For this review, take the finished solid that the model builds, in its own axes (mm). A direction names the side the tool comes from. Coordinates: 2 decimals unless noted, no trailing zeros. Loops run counter-clockwise (first coordinate to the right, second up) from the corner with the lowest first, then second, coordinate; pieces in that order, holes last.
Autodesk Inventor part; units mm, degrees
ref_plane "YZ Plane" through (0, 0, 0) normal (1, 0, 0) x (0, 1, 0)
ref_plane "XZ Plane" through (0, 0, 0) normal (0, 1, 0) x (-1, 0, 0)
ref_plane "XY Plane" through (0, 0, 0) normal (0, 0, 1) x (1, 0, 0)
sketch "スケッチ1" plane through (0, 0, 0) normal (1, 0, 0) x (0, 1, 0)
  circle A0 centre (0, 0) radius 5
  line L0 (5, 24) -> (-10, 24)
  line L1 (-10, 24) -> (-10, 9)
  line L2 (-10, 9) -> (5, 9)
  line L3 (5, 9) -> (5, 24)
  line L4 (-10, 9) -> (-15, 9)
  line L5 (-15, 9) -> (-15, -9)
  line L6 (-15, -9) -> (-10, -9)
  line L7 (-10, -9) -> (-10, 9)
  line L8 (-10, 9) -> (1.724, 4.6934)
  line L9 (1.724, -4.6934) -> (-10, -9)
  circle A1 centre (0, 0) radius 1.6
  line L10 (-10, 9) -> (-5, 9)
  line L11 (-5, 9) -> (-5, -9)
  line L12 (-5, -9) -> (-10, -9)
  line L13 (-10, -9) -> (-10, 9)
  line L14 (-5, 9) -> (2.6415, 4.2453)
  line L15 (-5, -9) -> (2.6415, -4.2453)
  line L16 (-5, 7) -> (-10, 7)
  line L17 (-5, 7) -> (1.6216, 4.7297)
  dimension "d0" = 10
  dimension "d1" = 15
  dimension "d2" = 15
  dimension "d3" = 5
  dimension "d5" = 18
  dimension "d6" = 3.2
  dimension "d7" = 10
  dimension "d8" = 9
  dimension "d11" = 5
  dimension "d12" = 18
  dimension "d29" = 2
extrude "押し出し2" add sketch "スケッチ1" along normal blind 5 contours A0 | A0 L8 L11 L14 | L15 L11 L9 A0 | L11 L8 L2 | L9 L11 A0 | L12 L9 L11 | L17 L11 L8 | A0 L11 L17 | L8 L11 L16 L7 | L11 L9 L7 L16
fillet "フィレット1" radius 2 2 edges at (2.5, -5, -9) (2.5, -5, 9)
sketch "スケッチ2" plane through (0, -10, -9) normal (0, -1, 0) x (1, 0, 0)
  circle A0 centre (2.5, 3.5) radius 1.25
  line L0 (0, 0) -> (5, 0)
  line L1 (0, 18) -> (0, 0)
  circle A1 centre (2.5, 10.5) radius 1.25
  point P0 (0, 9)
  dimension "d16" = 2.5
  dimension "d17" = 3.5
  dimension "d18" = 2.5
  dimension "d19" = 2.5
  dimension "d20" = 2.5
  dimension "d21" = 7
hole "穴1" at (2.5, -10, 1.5) at (2.5, -10, -5.5) direction (0, 1, 0) diameter 2.5 depth 5 tip angle 118
extrude "押し出し3" cut sketch "スケッチ1" along normal blind 10 contours A0 L8 L11 L14 | L11 L8 L2 | L17 L11 L8 | L8 L11 L16 L7
fillet "フィレット2" radius 2 1 edges at (2.5, -5, 7)
equation "\"d12\" = d5"
equation "\"d18\" = d16"
equation "\"d20\" = d18"
properties part number "belt_liner_v5_Plate_10" material "アルミニウム 6061"
Q1. Machinability: for faces 1 (the face through (2.45, -7.46, -4.25)), 2 (the face through (2, -8, 7)), which of the approach directions +Z, -Z, +X, -X, +Y, -Y give a long, thin tool a straight path to every point of the face, cutting with its end or side? Answer none if there is none.
Q2. Consider section A-A (z = 0). State the section outline as (x, y) points, then the cut area to 3 significant figures.
Q3. Consider section D-D (y = 0). State the section outline as (x, z) points.
Q4. For pin 1 Ø2 at (x, y) = (3, -3) entering from -Z; pin 2 Ø2 at (x, z) = (2.5, -5.5) entering from +Y; pin 3 Ø1 at (x, y) = (4.5, 3) entering from -Z; pin 4 Ø3 at (y, z) = (0, 0) entering from +X, all flat-tipped, find the tip position at first contact; note any pin that passes through.
Q5. Consider section B-B (x = 4.1). State the section outline as (y, z) points.
Q6. Wall thickness on probe 1 along Z at (x, y) = (2.5, -7.95); probe 2 along X at (y, z) = (-8, -5.5); probe 3 along Z at (x, y) = (3.2, -8): over which ranges is each line inside the solid? List them lowest first.
Q7. The part is to be moulded in two halves that separate along Y. For faces 3 (the face through (2.465, -0.987, -6.503)), 4 (the face through (2.12, -7.46, 0.31)), 5 (the face through (2.46, -1.27, 0.97)), say which applies: +Y half, -Y half, draft (parallel to the pull), parting line (faces both ways), or undercut.
Q8. Consider section C-C (y = -6). State the section outline as (x, z) points.
Model answer:
1. face 1: -Y
1. face 2: +Z, +X, -X, +Y, -Y
2. outline: (0, -10) - (5, -10) - (5, -1.6) - (0, -1.6) - close; (0, 1.6) - (5, 1.6) - (5, 5) - (0, 5) - close
2. area: 59.0 mm2
3. outline: (0, -5.89) - (5, -5.89) - (5, -1.6) - (0, -1.6) - close; (0, 1.6) - (5, 1.6) - (5, 5.29) - (0, 5.29) - close
4. pin 1: stops at z = -8.38
4. pin 2: stops at y = 2.23
4. pin 3: stops at z = -4.33
4. pin 4: passes through
5. outline: (-10, -9) - (-5.57, -9) arc R2 ccw to (-4.51, -8.7) - (2.64, -4.25) arc R5 ccw to (1.62, 4.73) - (-4.68, 6.89) arc R2 ccw to (-5.33, 7) - (-10, 7) - close; hole circle Ø3.2 at (0, 0)
6. probe 1: z = -9 to -6.75, -4.25 to 0.25, 2.75 to 7
6. probe 2: x = 0 to 1.25, 3.75 to 5
6. probe 3: z = -9 to -6.54, -4.46 to 0.46, 2.54 to 7
7. face 3: +Y half
7. face 4: draft
7. face 5: undercut
8. outline: (0, -9) - (5, -9) - (5, 7) - (0, 7) - close; hole circle Ø2.5 at (2.5, -5.5); hole circle Ø2.5 at (2.5, 1.5)
